For this review, take the finished solid that the model builds, in its own axes (mm). A direction names the side the tool comes from. Give positions to 0.01 mm unless a question says otherwise; leave off trailing zeros. Loops run counter-clockwise (first coordinate to the right, second up) from the corner with the lowest first, then second, coordinate; pieces in that order, holes last. Notation, with made-up numbers: (1, -8) -> (47, -8) arc R9 cw to (47, 0) -> close; hole circle Ø4 at (81.25, 78.25). An arc over 180 degrees is marked (long way). One line per question, with ' | ' between items. Start each with the question number.
(1) Consider section D-D (x = 0). Write out the cut boundary in (y, z) (3 decimals).
(2) Wall thickness on probe 1 along Y at (x, z) = (0, -4) (3 decimals); probe 2 along X at (y, z) = (-55, 1.5); probe 3 along Z at (x, y) = (6.5, -15): over which ranges is each line inside the solid? List them lowest first.
(3) Draft analysis for pull direction X (two halves, no side actions). For faces 1 (the flat face through (15.875, -63, 0)), 2 (the flat face through (0, 0, -22.225)), 3 (the cylindrical face through (-6.923, -55.337, -0.044)), state which applies: +X half, -X half, draft (parallel to the pull), parting line (faces both ways), or undercut.
(4) Tool access review of faces 4 (the flat face through (6.35, -42, 0)), 5 (the flat face through (0, 0, -12.954)), 6 (the flat face through (19.562, -38.538, 0.044)), 7 (the flat face through (-17, 10, 9.525)): name each direction out of +Z, -Z, +X, -X, +Y, -Y from which nothing blocks a thin tool from reaching the whole face with its end or side.
(5) Consider section B-B (z = 1.5). Write out the cut boundary in (x, y) (3 decimals).
(6) Consider section A-A (y = -40). Write out the cut boundary in (x, z) (3 decimals), and give its area (3 significant figures).
(7) Consider section C-C (y = 0). Write out the cut boundary in (x, z) (3 decimals), and give its area (3 significant figures).
(8) Insertion check: P1, Ø5, axis at y = -37, z = 5, coming from the +X side; P2, Ø5, axis at x = -15, z = 0, coming from the +Y side; P3, Ø5, axis at x = -20.5, z = 1, coming from the -Y side (3 decimals); P4, Ø19, axis at x = 9.5, y = 6.5, coming from the +Z side (3 decimals). Each pin has a flat end and moves straight along its axis. Give the tip position at first contact, or say it passes through.
from build123d import *

# Parameters (mm, degrees)
BOSS_EXTRUDE1_DEPTH = 3.175
CUT_EXTRUDE1_DEPTH  = 6.35


with BuildPart() as part:
    # Sketch2 → Boss-Extrude1 (new, symmetric)
    with BuildSketch(Plane.XY):
        Polygon((-9.235964967, 0), (9.235964967, 0), (25.4, -60.325), (15.875, -60.325), (15.875, -66.675), (-15.875, -66.675), (-15.875, -60.325), (-25.4, -60.325), align=None)
    extrude(amount=BOSS_EXTRUDE1_DEPTH, both=True)

    # Sketch3 → Revolve1 (revolve)
    with BuildSketch(Plane(origin=(0, 0, 0), x_dir=(0, 0, -1), z_dir=(1, 0, 0)), mode=Mode.PRIVATE) as revolve1_sk:
        with BuildLine():
            Line((22.225, 0), (22.225, 15.875))
            ThreePointArc((22.225, 15.875), (20.365128061, 20.365128061), (15.875, 22.225))
            Line((15.875, 22.225), (-9.525, 22.225))
            Line((-9.525, 22.225), (-9.525, 0))
            Line((-9.525, 0), (0, 0))
            Line((0, 0), (22.225, 0))
        make_face()
    revolve(revolve1_sk.sketch.rotate(Axis((0, 0, 0), (0, 0, -1)), 90), axis=Axis((0, 0, 0), (0, 0, -1)))

    # Sketch5 → Cut-Revolve1 (revolve, cut)
    with BuildSketch(Plane(origin=(0, 0, 0), x_dir=(0, 0, -1), z_dir=(1, 0, 0)), mode=Mode.PRIVATE) as cut_revolve1_sk:
        Polygon((-9.525, 19.177), (-6.35, 19.177), (-6.35, 4.826), (12.954, 4.826), (12.954, 0), (-9.525, 0), align=None)
    revolve(cut_revolve1_sk.sketch.rotate(Axis((0, 0, 9.525), (0, 0, -1)), 90), axis=Axis((0, 0, 9.525), (0, 0, -1)), mode=Mode.SUBTRACT)

    # Sketch6 → Cut-Extrude1 (cut)
    with BuildSketch(Plane(origin=(0, 0, -3.175), x_dir=(-1, 0, 0), z_dir=(0, 0, -1))):
        with BuildLine():
            Line((-13.983942054, -29.986949719), (-20.279408331, -53.481949719))
            ThreePointArc((-20.279408331, -53.481949719), (-19.950657745, -55.134690522), (-18.439319632, -55.88))
            Line((-18.439319632, -55.88), (-8.255, -55.88))
            ThreePointArc((-8.255, -55.88), (-6.907961582, -55.322038418), (-6.35, -53.975))
            Line((-6.35, -53.975), (-6.35, -30.48))
            ThreePointArc((-6.35, -30.48), (-6.907961582, -29.132961582), (-8.255, -28.575))
            Line((-8.255, -28.575), (-12.143853355, -28.575))
            ThreePointArc((-12.143853355, -28.575), (-13.303543878, -28.968661887), (-13.983942054, -29.986949719))
        make_face()
        with BuildLine():
            Line((8.255, -28.575), (12.143853355, -28.575))
            ThreePointArc((12.143853355, -28.575), (13.303543878, -28.968661887), (13.983942054, -29.986949719))
            Line((13.983942054, -29.986949719), (20.279408331, -53.481949719))
            ThreePointArc((20.279408331, -53.481949719), (19.950657745, -55.134690522), (18.439319632, -55.88))
            Line((18.439319632, -55.88), (8.255, -55.88))
            ThreePointArc((8.255, -55.88), (6.907961582, -55.322038418), (6.35, -53.975))
            Line((6.35, -53.975), (6.35, -30.48))
            ThreePointArc((6.35, -30.48), (6.907961582, -29.132961582), (8.255, -28.575))
        make_face()
    extrude(amount=-CUT_EXTRUDE1_DEPTH, mode=Mode.SUBTRACT)


solid = part.part
A:
1) outline: (-66.675, -3.175) -> (-22.225, -3.175) -> (-22.225, -15.875) arc R6.35 ccw to (-15.875, -22.225) -> (15.875, -22.225) arc R6.35 ccw to (22.225, -15.875) -> (22.225, 9.525) -> (19.177, 9.525) -> (19.177, 6.35) -> (4.826, 6.35) -> (4.826, -12.954) -> (-4.826, -12.954) -> (-4.826, 6.35) -> (-19.177, 6.35) -> (-19.177, 9.525) -> (-22.225, 9.525) -> (-22.225, 3.175) -> (-66.675, 3.175) -> close
2) probe 1: y = -22.225 to -4.826, 4.826 to 22.225 | probe 2: x = -23.97 to -20.05, -6.65 to 6.65, 20.05 to 23.97 | probe 3: z = -22.21 to 6.35
3) face 1: +X half | face 2: draft | face 3: undercut
4) face 4: +Z, -Z | face 5: +Z | face 6: +Z, -Z, +X | face 7: +Z, +X, -X, +Y, -Y
5) outline: (-25.4, -60.325) -> (-15.875, -60.325) -> (-15.875, -66.675) -> (15.875, -66.675) -> (15.875, -60.325) -> (25.4, -60.325) -> (13.886, -17.353) arc R22.225 ccw (long way) to (-13.886, -17.353) -> close; hole (-20.279, -53.482) arc R1.905 ccw to (-18.439, -55.88) -> (-8.255, -55.88) arc R1.905 ccw to (-6.35, -53.975) -> (-6.35, -30.48) arc R1.905 ccw to (-8.255, -28.575) -> (-12.144, -28.575) arc R1.905 ccw to (-13.984, -29.987) -> close; hole circle Ø9.652 at (0, 0); hole (6.35, -53.975) arc R1.905 ccw to (8.255, -55.88) -> (18.439, -55.88) arc R1.905 ccw to (20.279, -53.482) -> (13.984, -29.987) arc R1.905 ccw to (12.144, -28.575) -> (8.255, -28.575) arc R1.905 ccw to (6.35, -30.48) -> close
6) outline: (-19.954, -3.175) -> (-16.667, -3.175) -> (-16.667, 3.175) -> (-19.954, 3.175) -> close; (-6.35, -3.175) -> (6.35, -3.175) -> (6.35, 3.175) -> (-6.35, 3.175) -> close; (16.667, -3.175) -> (19.954, -3.175) -> (19.954, 3.175) -> (16.667, 3.175) -> close | area: 122 mm^2
7) outline: (-22.225, -15.875) arc R6.35 ccw to (-15.875, -22.225) -> (15.875, -22.225) arc R6.35 ccw to (22.225, -15.875) -> (22.225, 9.525) -> (19.177, 9.525) -> (19.177, 6.35) -> (4.826, 6.35) -> (4.826, -12.954) -> (-4.826, -12.954) -> (-4.826, 6.35) -> (-19.177, 6.35) -> (-19.177, 9.525) -> (-22.225, 9.525) -> close | area: 1,090 mm^2
8) P1: stops at x = 19.61 | P2: stops at y = 18.38 | P3: stops at y = -60.325 | P4: stops at z = 9.525
